Design review of the part shown in the three views and the two pictorial views. Dimensions are in mm from the part's minimum x, y and z. A direction names the side the tool comes from. Give positions to 0.01 mm unless a question says otherwise; leave off trailing zeros. Loops run counter-clockwise (first coordinate to the right, second up) from the corner with the lowest first, then second, coordinate; pieces in that order, holes last. Notation, with made-up numbers: (-9.5, 55.5) - (-5.5, 55.5) arc R23 ccw to (-5.5, 92.5) - close; hole circle Ø9 at (-28, 44.25). An arc over 180 degrees is marked (long way). Answer as a JSON object with one key per item and string values.
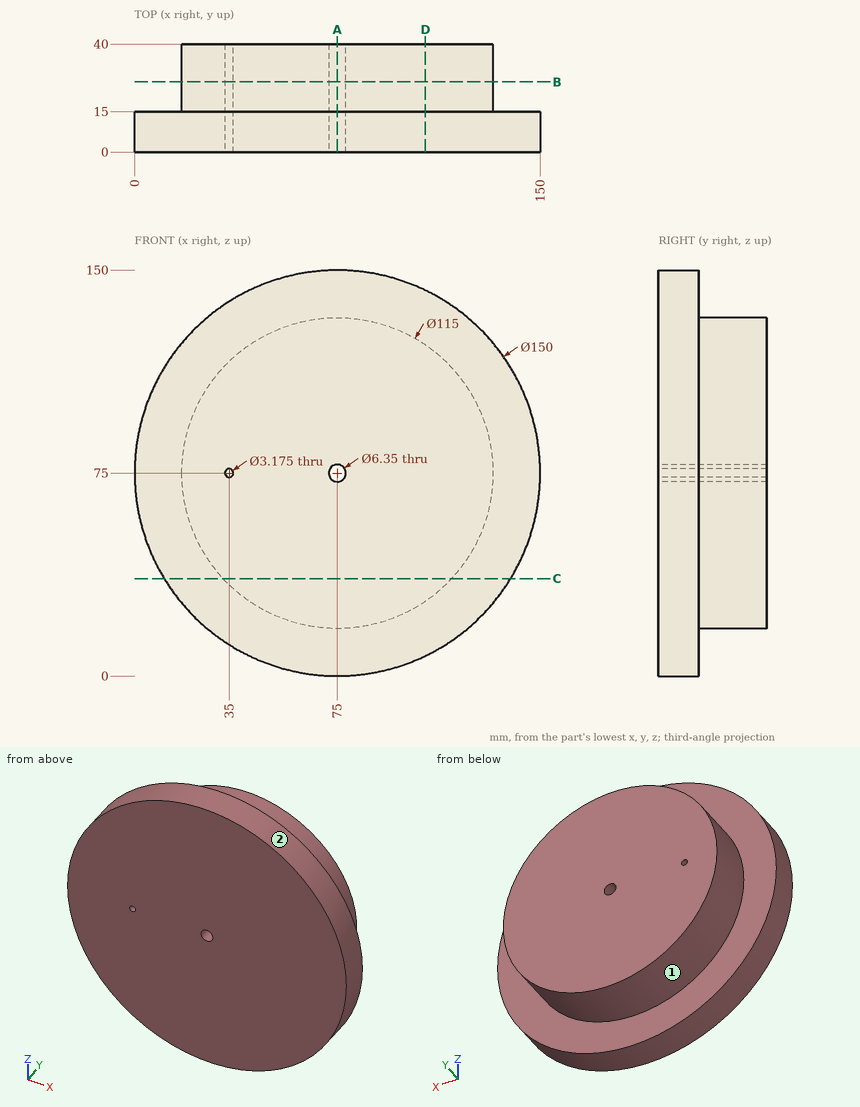
Q1. Consider section A-A, the plane x = 75. State the section outline as (y, z) points (3 decimals).
Results:
{"outline": "(0, 0) - (15, 0) - (15, 17.5) - (40, 17.5) - (40, 71.825) - (0, 71.825) - close; (0, 78.175) - (40, 78.175) - (40, 132.5) - (15, 132.5) - (15, 150) - (0, 150) - close"}
Q2. For the marked faces 1 and 2, list the 3-axis set-ups (+Z, -Z, +X, -X, +Y, -Y) from which the entire face can be reached by the end or side of a thin tool; tool diameter is ignored.
Results:
{"face 1": "+Y", "face 2": "+Y, -Y"}
Q3. Clearance check with flat-ended pins moving along their axes: pin 1 Ø4 at (x, z) = (17.5, 31.5) entering from -Y; pin 2 Ø4 at (y, z) = (36, 96) entering from -X; pin 3 Ø6 at (x, y) = (68.5, 31) entering from -Z; pin 4 Ø5 at (y, z) = (26, 103.5) entering from -X. State where each tip first meets the part, or that it passes through.
Results:
{"pin 1": "stops at y = 0", "pin 2": "stops at x = 20.73", "pin 3": "stops at z = 17.61", "pin 4": "stops at x = 23.71"}
Q4. Consider section D-D, the plane x = 107.5. State the section outline as (y, z) points.
Results:
{"outline": "(0, 7.41) - (15, 7.41) - (15, 27.57) - (40, 27.57) - (40, 122.43) - (15, 122.43) - (15, 142.59) - (0, 142.59) - close"}
Q5. Consider section B-B, the plane y = 26. State how many separate pieces and enclosed holes the cut face has, plus the area to 3 significant figures.
Results:
{"separate pieces": "1", "enclosed holes": "2", "area": "10,300 mm^2"}
Q6. Consider section C-C, the plane z = 36. State the section outline as (x, y) points, plus the area to 3 significant figures.
Results:
{"outline": "(10.94, 0) - (139.06, 0) - (139.06, 15) - (117.25, 15) - (117.25, 40) - (32.75, 40) - (32.75, 15) - (10.94, 15) - close", "area": "4,030 mm^2"}
Q7. To check wall thickness, follow probe 1 along Z at (x, y) = (75, 21) (3 decimals); probe 2 along Z at (x, y) = (75, 14) (3 decimals); probe 3 along Y at (x, z) = (131, 47). State the ranges of each line that lie inside material, in increasing order. Write a range as [from, to].
Results:
{"probe 1": "z = [17.5, 71.825], [78.175, 132.5]", "probe 2": "z = [0, 71.825], [78.175, 150]", "probe 3": "y = [0, 15]"}
